from build123d import *

# Parameters (mm, degrees)
SKETCH1_R           = 30
SKETCH1_R_2         = 10
SKETCH1_R_3         = 2.1
BOSS_EXTRUDE1_DEPTH = 10.35
SKETCH2_R           = 14.3875
CUT_EXTRUDE2_DEPTH  = 8


with BuildPart() as part:
    # Sketch1 → Boss-Extrude1 (new body)
    with BuildSketch(Plane(origin=(0, 0, 0), x_dir=(1, 0, 0), z_dir=(0, 1, 0))):
        with Locations(Location((0, 0, 0), (0, 0, 270))):
            Circle(SKETCH1_R)
        with Locations(Location((0, 0, 0), (0, 0, 270))):
            Circle(SKETCH1_R_2, mode=Mode.SUBTRACT)
        with Locations(Location((0, 25, 0), (0, 0, 270))):
            Circle(SKETCH1_R_3, mode=Mode.SUBTRACT)
        with Locations(Location((25, 0, 0), (0, 0, 270))):
            Circle(SKETCH1_R_3, mode=Mode.SUBTRACT)
        with Locations(Location((0, -25, 0), (0, 0, 270))):
            Circle(SKETCH1_R_3, mode=Mode.SUBTRACT)
        with Locations(Location((-25, 0, 0), (0, 0, 270))):
            Circle(SKETCH1_R_3, mode=Mode.SUBTRACT)
    extrude(amount=BOSS_EXTRUDE1_DEPTH)

    # Sketch2 → Cut-Extrude2 (cut)
    with BuildSketch(Plane(origin=(0, 0, 0), x_dir=(1, 0, 0), z_dir=(0, 1, 0))):
        with Locations(Location((0, 0, 0), (0, 0, 270))):
            Circle(SKETCH2_R)
    extrude(amount=CUT_EXTRUDE2_DEPTH, mode=Mode.SUBTRACT)


solid = part.part
Geometry: final body of the model. Coordinates: model frame, mm. A direction names the side the tool comes from. Coordinates: 2 decimals unless noted, no trailing zeros. Loops run counter-clockwise (first coordinate to the right, second up) from the corner with the lowest first, then second, coordinate; pieces in that order, holes last. Notation, with made-up numbers: M 79.5,55 L 91.5,55 A14 ccw 91.5,62 Z; hole C 18.25,-38.5 d2. An arc over 180 degrees is marked long. One line per item, written item: value. Start each with the question number.
1) Reachability of faces 1 (the cylindrical face through (26.77, 5.1, 1.13)), 2 (the flat face through (-3, 8, -10)) from +Z, -Z, +X, -X, +Y, -Y: full face, straight path, thin tool, end or side. Return the list, or none.
2) Pin query (flat end, axial travel): P1, Ø6, axis at y = 1.5, z = -14.5, coming from the +X side; P2, Ø4, axis at x = 3.5, y = 2, coming from the -Z side; P3, Ø1, axis at x = -6.5, y = 3.5, coming from the -Z side. Return the tip coordinate at first contact, or that it passes through.
3) Cut plane D-D (z = 7). Return loops of the section in (x, y).
4) Draft query along Z for faces 3 (the cylindrical face through (-23.23, 5.1, 1.13)), 4 (the cylindrical face through (1.32, 5.1, -29.97)), 5 (the flat face through (7, 0, 13)), 6 (the cylindrical face through (12.132, 3.944, 7.735)). Return one class per face: released by +Z, released by -Z, zero draft, split by the parting line, or undercut.
5) Cut plane A-A (x = 0). Return loops of the section in (y, z), then the cut area to 3 significant figures.
6) Cut plane B-B (z = 0). Return loops of the section in (x, y), then the cut area to 3 significant figures.
7) Material intervals for L1, parallel to X at y = 7.25, z = 0; L2, parallel to X at y = 5.5, z = -1; L3, parallel to X at y = 6.25, z = 6, sorted ascending. Write a range as from..to.
8) Cut plane C-C (y = 6.5). Return loops of the section in (x, z) (1 decimal).
Evaluation:
1. face 1: +Y, -Y
1. face 2: -Y
2. P1: x = 27.71
2. P2: z = -29.96
2. P3: z = -29.39
3. outline: M -29.17,0 L -12.57,0 L -12.57,8 L -7.14,8 L -7.14,10.35 L -29.17,10.35 Z; M 7.14,8 L 12.57,8 L 12.57,0 L 29.17,0 L 29.17,10.35 L 7.14,10.35 Z
4. face 3: undercut
4. face 4: split by the parting line
4. face 5: zero draft
4. face 6: undercut
5. outline: M 0,-30 L 10.35,-30 L 10.35,-27.1 L 0,-27.1 Z; M 0,-22.9 L 10.35,-22.9 L 10.35,-10 L 8,-10 L 8,-14.39 L 0,-14.39 Z; M 0,14.39 L 8,14.39 L 8,10 L 10.35,10 L 10.35,22.9 L 0,22.9 Z; M 0,27.1 L 10.35,27.1 L 10.35,30 L 0,30 Z
5. area: 257 mm^2
6. outline: M -30,0 L -27.1,0 L -27.1,10.35 L -30,10.35 Z; M -22.9,0 L -14.39,0 L -14.39,8 L -10,8 L -10,10.35 L -22.9,10.35 Z; M 10,8 L 14.39,8 L 14.39,0 L 22.9,0 L 22.9,10.35 L 10,10.35 Z; M 27.1,0 L 30,0 L 30,10.35 L 27.1,10.35 Z
6. area: 257 mm^2
7. L1: -30..-27.1, -22.9..-14.39, 14.39..22.9, 27.1..30
7. L2: -29.98..-26.85, -23.15..-14.35, 14.35..23.15, 26.85..29.98
7. L3: -29.39..-13.08, 13.08..29.39
8. outline: C 0,0 d60; hole C -25,0 d4.2; hole C 0,0 d28.8; hole C 0,-25 d4.2; hole C 0,25 d4.2; hole C 25,0 d4.2
